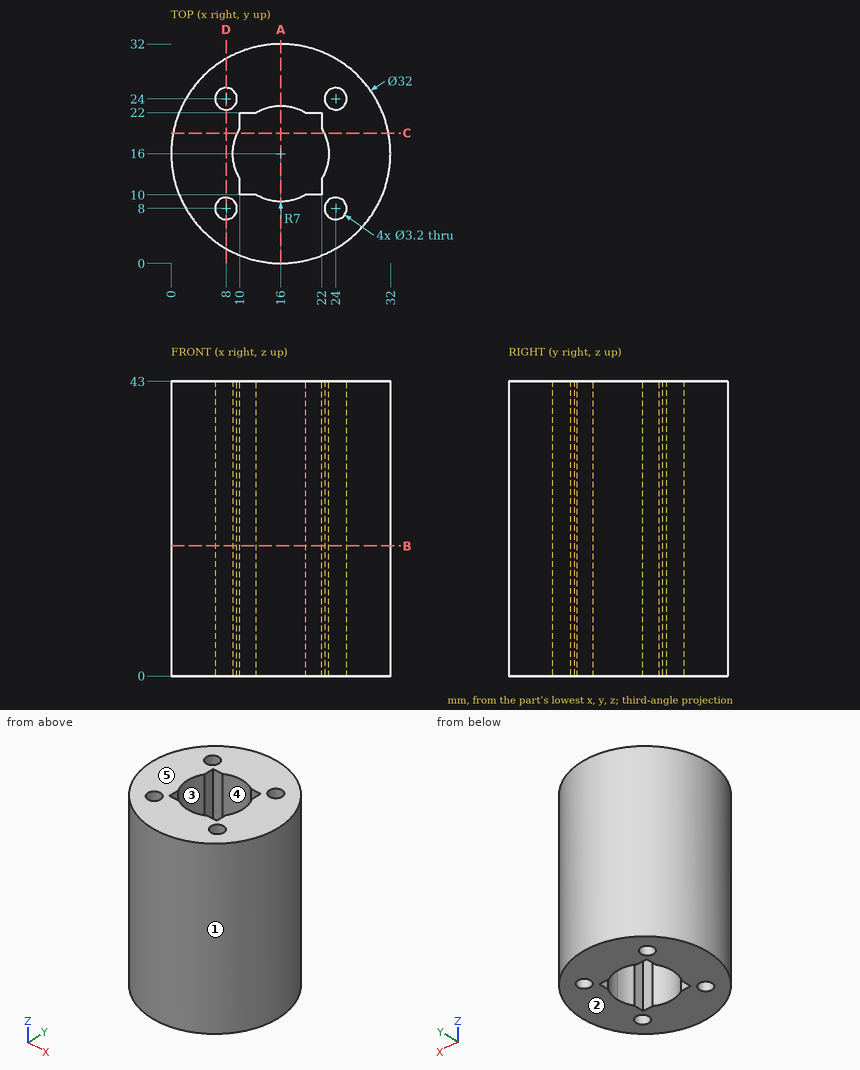
Verification items for this drawing (mm, ordinates from the low corner). A direction names the side the tool comes from. Coordinates: 2 decimals unless noted, no trailing zeros. Write each loop counter-clockwise with the first axis right and the second up, starting at its lowest first coordinate (ties: lowest second). Pieces come first, ordered by that corner, then holes. Notation, with made-up numbers: M 40.25,59 L 96.25,59 A10 cw 96.25,71 Z; hole C 82.25,88 d11. An arc over 180 degrees is marked long. Answer as a JSON object with one key per item and string values.
1. Section check C-C, the plane y = 19. Enter the section's corners in (x, z), plus the area to 3 significant figures.
Answers below:
{"outline": "M 0.28,0 L 9.68,0 L 9.68,43 L 0.28,43 Z; M 22.32,0 L 31.72,0 L 31.72,43 L 22.32,43 Z", "area": "808 mm²"}
2. Draft check along Y on the marked faces 1, 2 and 3. Enter one of: released by +Y, released by -Y, zero draft, split by the parting line, or undercut.
Answers below:
{"face 1": "split by the parting line", "face 2": "zero draft", "face 3": "undercut"}
3. Section check D-D, the plane x = 8. Enter the section's corners in (y, z).
Answers below:
{"outline": "M 2.14,0 L 6.4,0 L 6.4,43 L 2.14,43 Z; M 9.6,0 L 22.4,0 L 22.4,43 L 9.6,43 Z; M 25.6,0 L 29.86,0 L 29.86,43 L 25.6,43 Z"}
4. Section check B-B, the plane z = 19. Enter the section's corners in (x, y).
Answers below:
{"outline": "C 16,16 d32; hole C 8,8 d3.2; hole C 8,24 d3.2; hole M 10,10 L 12.39,10 A7 ccw 19.61,10 L 22,10 L 22,12.39 A7 ccw 22,19.61 L 22,22 L 19.61,22 A7 ccw 12.39,22 L 10,22 L 10,19.61 A7 ccw 10,12.39 Z; hole C 24,8 d3.2; hole C 24,24 d3.2"}
5. Go/stop test with flat-tipped pins: pin 1 Ø2.5 at (x, z) = (20.5, 31.5) entering from +Y; pin 2 Ø1.9 at (x, z) = (11.5, 25) entering from -Y; pin 3 Ø1.2 at (x, z) = (21, 14) entering from -Y; pin 4 Ø1.9 at (x, y) = (8, 8) entering from -Z. Record where each tip stops, or that it passes through.
Answers below:
{"pin 1": "stops at y = 31.67", "pin 2": "stops at y = 0.4", "pin 3": "stops at y = 0.62", "pin 4": "passes through"}
6. Tool access check on the marked faces 4 and 5. Record the directions out of +Z, -Z, +X, -X, +Y, -Y that give a thin tool (end or side, any length) a straight path to the whole face; none if there is none.
Answers below:
{"face 4": "+Z, -Z", "face 5": "+Z, +X, -X, +Y, -Y"}
7. Section check A-A, the plane x = 16. Enter the section's corners in (y, z), plus the area to 3 significant figures.
Answers below:
{"outline": "M 0,0 L 9,0 L 9,43 L 0,43 Z; M 23,0 L 32,0 L 32,43 L 23,43 Z", "area": "774 mm²"}
8. Scan lines: L1, parallel to Y at x = 16, z = 13; L2, parallel to Y at x = 8, z = 21; L3, parallel to Y at x = 25, z = 3. Record each from-to range of solid material in increasing order.
Answers below:
{"L1": "y = 0 to 9, 23 to 32", "L2": "y = 2.14 to 6.4, 9.6 to 22.4, 25.6 to 29.86", "L3": "y = 2.77 to 6.75, 9.25 to 22.75, 25.25 to 29.23"}
